Check sheet for the modelled part. Datum: model origin and axes. Units: mm. Round coordinates to 2 decimals unless told otherwise and drop trailing zeros. Loops run counter-clockwise (first coordinate to the right, second up) from the corner with the lowest first, then second, coordinate; pieces in that order, holes last. Notation, with made-up numbers: (52.5, 66.25) -> (78.5, 66.25) arc R18 cw to (78.5, 75.25) -> close; hole circle Ø9 at (24, 72.5). An arc over 180 degrees is marked (long way). Return JSON: item names as keys, results as strings.
from build123d import *

# Parameters (mm, degrees)
ESQUISSE1_R        = 1
BOSS_EXTRU_2_DEPTH = 2


with BuildPart() as part:
    # Esquisse1 → Boss.-Extru.2 (new body)
    with BuildSketch(Plane(origin=(0, 0, 0), x_dir=(1, 0, 0), z_dir=(0, 1, 0))):
        with BuildLine():
            Line((0, 103), (127, 103))
            Line((127, 103), (3, -5.196152423))
            ThreePointArc((3, -5.196152423), (-3, -5.196152423), (-6, 0))
            Line((-6, 0), (0, 103))
        make_face()
        Circle(ESQUISSE1_R, mode=Mode.SUBTRACT)
    extrude(amount=BOSS_EXTRU_2_DEPTH)


solid = part.part
Q1. Section check C-C (x = 103). Record the boundary of the cut face in (y, z), then the cut area to 3 significant figures.
Results list:
{"outline": "(0, -103) -> (2, -103) -> (2, -82.06) -> (0, -82.06) -> close", "area": "41.9 mm^2"}
Q2. Section check B-B (z = -73). Record the boundary of the cut face in (x, y), then the cut area to 3 significant figures.
Results list:
{"outline": "(-1.75, 0) -> (92.62, 0) -> (92.62, 2) -> (-1.75, 2) -> close", "area": "189 mm^2"}
Q3. Section check A-A (y = 0.8). Record the boundary of the cut face in (x, z), then the cut area to 3 significant figures.
Results list:
{"outline": "(-6, 0) -> (0, -103) -> (127, -103) -> (3, 5.2) arc R6 ccw to start; hole circle Ø2 at (0, 0)", "area": "7,370 mm^2"}
Q4. Material ranges on line 1 (X direction, y = 0.9, z = 0); line 2 (Z direction, x = 68, y = 0.6); line 3 (X direction, y = 1.05, z = -92.5), recorded low to high.
Results list:
{"line 1": "-6 to -1, 1 to 8.96", "line 2": "-103 to -51.52", "line 3": "-0.61 to 114.97"}
